Geometry check sheet. Reference: the model listing, model coordinates, mm. Give positions to 0.01 mm unless a question says otherwise; leave off trailing zeros. Order: outer loops, then holes, each group sorted by start corner. A loop starts at its lowest first (then second) coordinate and runs counter-clockwise, first axis right, second up.
from build123d import *

# Parameters (mm, degrees)
SKETCH1_W           = 155
SKETCH1_H           = 110
BOSS_EXTRUDE1_DEPTH = 80
SKETCH2_W           = 151
SKETCH2_H           = 106
CUT_EXTRUDE1_DEPTH  = 78
SKETCH3_R           = 2.5
CUT_EXTRUDE2_DEPTH  = 2
SKETCH7_R           = 1.6
CUT_EXTRUDE7_DEPTH  = 2
SKETCH4_W           = 27.5
SKETCH4_H           = 46.8
CUT_EXTRUDE8_DEPTH  = 2
SKETCH8_W           = 4
SKETCH8_H           = 53
CUT_EXTRUDE9_DEPTH  = 2
SKETCH9_W           = 14
SKETCH9_H           = 14
CUT_EXTRUDE10_DEPTH = 2
SKETCH10_W          = 25.2
SKETCH10_H          = 71.2
SKETCH10_R          = 1.25
CUT_EXTRUDE12_DEPTH = 2
SKETCH11_R          = 2.5
SKETCH11_R_2        = 4.5
CUT_EXTRUDE13_DEPTH = 2
SKETCH12_W          = 153
SKETCH12_H          = 110
CUT_EXTRUDE14_DEPTH = 80


with BuildPart() as part:
    # Sketch1 → Boss-Extrude1 (new body)
    with BuildSketch(Plane.XY):
        with Locations((77.5, 55)):
            Rectangle(SKETCH1_W, SKETCH1_H)
    extrude(amount=BOSS_EXTRUDE1_DEPTH)

    # Sketch2 → Cut-Extrude1 (cut)
    with BuildSketch(Plane.XY.offset(80)):
        with Locations((77.5, 55)):
            Rectangle(SKETCH2_W, SKETCH2_H)
    extrude(amount=-CUT_EXTRUDE1_DEPTH, mode=Mode.SUBTRACT)

    # Sketch3 → Cut-Extrude2 (cut)
    with BuildSketch(Plane.XY.offset(2)):
        with Locations((145, 100.5)):
            Circle(SKETCH3_R)
        with Locations((145, 9.5)):
            Circle(SKETCH3_R)
        with Locations((10, 9.5)):
            Circle(SKETCH3_R)
        with Locations((10, 100.5)):
            Circle(SKETCH3_R)
    extrude(amount=-CUT_EXTRUDE2_DEPTH, mode=Mode.SUBTRACT)

    # Sketch7 → Cut-Extrude7 (cut)
    with BuildSketch(Plane(origin=(0, 110, 0), x_dir=(1, 0, 0), z_dir=(0, 1, 0))):
        with Locations((44.48, -20.14450396)):
            Circle(SKETCH7_R)
        with Locations((95.28, -17.14)):
            Circle(SKETCH7_R)
        with Locations((95.28, -62.86)):
            Circle(SKETCH7_R)
        with Locations((44.48, -47.62)):
            Circle(SKETCH7_R)
    extrude(amount=-CUT_EXTRUDE7_DEPTH, mode=Mode.SUBTRACT)

    # Sketch4 → Cut-Extrude8 (cut)
    with BuildSketch(Plane(origin=(155, 0, 0), x_dir=(0, 0, -1), z_dir=(1, 0, 0))):
        with Locations((-40, 82.5)):
            Rectangle(SKETCH4_W, SKETCH4_H)
    extrude(amount=-CUT_EXTRUDE8_DEPTH, mode=Mode.SUBTRACT)

    # Sketch8 → Cut-Extrude9 (cut)
    with BuildSketch(Plane(origin=(155, 0, 0), x_dir=(0, 0, -1), z_dir=(1, 0, 0))):
        with Locations((-68, 28.5)):
            Rectangle(SKETCH8_W, SKETCH8_H)
        with Locations((-76, 28.5)):
            Rectangle(SKETCH8_W, SKETCH8_H)
        with Locations((-60, 28.5)):
            Rectangle(SKETCH8_W, SKETCH8_H)
        with Locations((-52, 28.5)):
            Rectangle(SKETCH8_W, SKETCH8_H)
        with Locations((-44, 28.5)):
            Rectangle(SKETCH8_W, SKETCH8_H)
        with Locations((-36, 28.5)):
            Rectangle(SKETCH8_W, SKETCH8_H)
        with Locations((-28, 28.5)):
            Rectangle(SKETCH8_W, SKETCH8_H)
        with Locations((-20, 28.5)):
            Rectangle(SKETCH8_W, SKETCH8_H)
        with Locations((-12, 28.5)):
            Rectangle(SKETCH8_W, SKETCH8_H)
        with Locations((-4, 28.5)):
            Rectangle(SKETCH8_W, SKETCH8_H)
    extrude(amount=-CUT_EXTRUDE9_DEPTH, mode=Mode.SUBTRACT)

    # Sketch9 → Cut-Extrude10 (cut)
    with BuildSketch(Plane(origin=(0, 110, 0), x_dir=(1, 0, 0), z_dir=(0, 1, 0))):
        with Locations((120, -19)):
            Rectangle(SKETCH9_W, SKETCH9_H)
    extrude(amount=-CUT_EXTRUDE10_DEPTH, mode=Mode.SUBTRACT)

    # Sketch10 → Cut-Extrude12 (cut)
    with BuildSketch(Plane.ZY):
        with Locations((58, 55)):
            Rectangle(SKETCH10_W, SKETCH10_H)
        with Locations((42.5, 92.5)):
            Circle(SKETCH10_R)
        with Locations((73.5, 92.5)):
            Circle(SKETCH10_R)
        with Locations((42.5, 17.5)):
            Circle(SKETCH10_R)
        with Locations((73.5, 17.5)):
            Circle(SKETCH10_R)
    extrude(amount=-CUT_EXTRUDE12_DEPTH, mode=Mode.SUBTRACT)

    # Sketch11 → Cut-Extrude13 (cut)
    with BuildSketch(Plane.ZY):
        with Locations((20, 55)):
            Circle(SKETCH11_R)
        with Locations((20, 40)):
            Circle(SKETCH11_R)
        with Locations((20, 25)):
            Circle(SKETCH11_R)
        with Locations((20, 82.5)):
            Circle(SKETCH11_R_2)
    extrude(amount=-CUT_EXTRUDE13_DEPTH, mode=Mode.SUBTRACT)

    # Sketch12 → Cut-Extrude14 (cut)
    with BuildSketch(Plane.XY.offset(80)):
        with Locations((76.5, 55)):
            Rectangle(SKETCH12_W, SKETCH12_H)
    extrude(amount=-CUT_EXTRUDE14_DEPTH, mode=Mode.SUBTRACT)


solid = part.part
Item 1: Scan lines: L1, parallel to Y at x = 153.35, z = 37.5; L2, parallel to Z at x = 153.5, y = 71.5; L3, parallel to Y at x = 154.55, z = 41.5. Record each from-to range of solid material in increasing order.
Reported:
L1: y = 0 to 2, 55 to 59.1, 105.9 to 110
L2: z = 0 to 26.25, 53.75 to 80
L3: y = 0 to 59.1, 105.9 to 110
Item 2: Sectioned sample at B-B (y = 7). Give the number of separate pieces and of enclosed holes in the cut face, and give its area (3 significant figures).
Reported:
separate pieces: 11
enclosed holes: 0
area: 80.0 mm2
Item 3: Sectioned sample at A-A (y = 70.5). Enter the section's corners in (x, z).
Reported:
outline: (153, 0) - (155, 0) - (155, 26.25) - (153, 26.25) - close; (153, 53.75) - (155, 53.75) - (155, 80) - (153, 80) - close
